Geometry: see drawing. Coordinates: mm, zero at the bounding-box minimum. A direction names the side the tool comes from. Give positions to 0.01 mm unless a question says otherwise; leave off trailing zeros. Loops run counter-clockwise (first coordinate to the right, second up) from the corner with the lowest first, then second, coordinate; pieces in that order, holes last. Notation, with made-up numbers: (-13, 81.25) -> (32, 81.25) arc R24 cw to (32, 99.25) -> close; hole circle Ø11 at (3.5, 56). An arc over 180 degrees is marked (long way). Return JSON: item names as keys, results as strings. Group by question number.
(1) Draft query along Y for the marked faces 3, 4, 5 and 6. Return one class per face: released by +Y, released by -Y, zero draft, split by the parting line, or undercut.
(2) Ray query, line 1 (Z direction, x = 25, y = 0.6); line 2 (X direction, y = 6, z = 10). Return the intervals inside material, ascending. Write a range as from..to.
(3) Pin query (flat end, axial travel): pin 1 (8 mm diameter, centred on y = 14.5, z = 18, fed in from +X); pin 2 (5.5 mm diameter, centred on x = 25, z = 21.25, fed in from -Y); pin 3 (12 mm diameter, centred on x = 4.5, y = 26, fed in from -Z); pin 4 (4.5 mm diameter, centred on x = 11, z = 21.25, fed in from +Y). Return the tip coordinate at first contact, or that it passes through.
(4) Cut plane B-B on x = 25. Return loops of the section in (y, z), then the cut area to 3 significant figures.
(5) Cut plane D-D on y = 17. Return loops of the section in (x, z), then the cut area to 3 significant figures.
(6) Cut plane A-A on z = 13.25. Return loops of the section in (x, y).
(7) Access query for the marked faces 1 and 2. Directions: +Z, -Z, +X, -X, +Y, -Y. A direction counts if a zero-diameter tool reaches every point of the face in a straight line with its end or side. Return the directions, or none.
(8) Cut plane C-C on x = 18. Return loops of the section in (y, z), then the cut area to 3 significant figures.
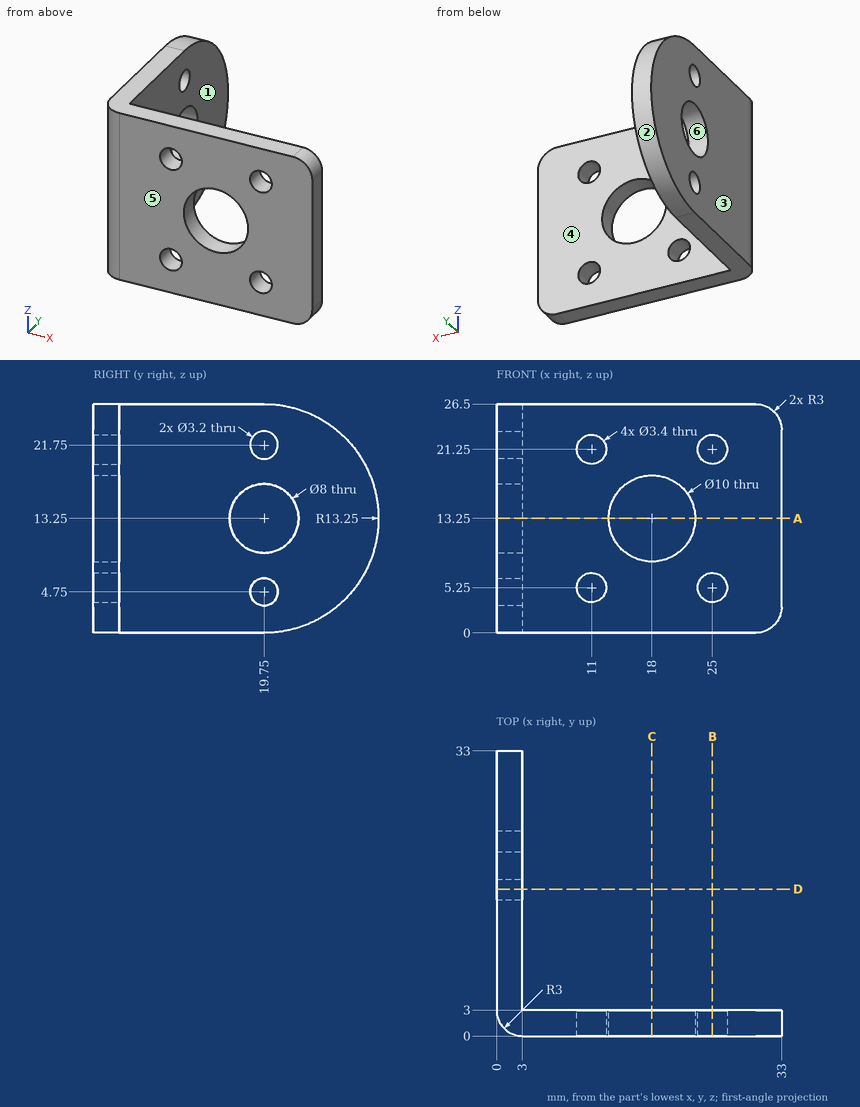
Answers:
{
 "1": {"face 3": "zero draft", "face 4": "released by +Y", "face 5": "released by -Y", "face 6": "undercut"},
 "2": {"line 1": "0..3.55, 6.95..19.55, 22.95..26.5", "line 2": "0..3"},
 "3": {"pin 1": "x = 3", "pin 2": "y = 0", "pin 3": "z = 0.01", "pin 4": "y = 3"},
 "4": {"outline": "(0, 0) -> (3, 0) -> (3, 3.55) -> (0, 3.55) -> close; (0, 6.95) -> (3, 6.95) -> (3, 19.55) -> (0, 19.55) -> close; (0, 22.95) -> (3, 22.95) -> (3, 26.5) -> (0, 26.5) -> close", "area": "59.1 mm²"},
 "5": {"outline": "(0, 0) -> (3, 0) -> (3, 10.35) -> (0, 10.35) -> close; (0, 16.15) -> (3, 16.15) -> (3, 26.5) -> (0, 26.5) -> close", "area": "62.1 mm²"},
 "6": {"outline": "(0, 3) arc R3 ccw to (3, 0) -> (13, 0) -> (13, 3) -> (3, 3) -> (3, 15.75) -> (0, 15.75) -> close; (0, 23.75) -> (3, 23.75) -> (3, 33) -> (0, 33) -> close; (23, 0) -> (33, 0) -> (33, 3) -> (23, 3) -> close"},
 "7": {"face 1": "+Z, -Z, +X, +Y", "face 2": "+X, -X, +Y"},
 "8": {"outline": "(0, 0) -> (3, 0) -> (3, 8.25) -> (0, 8.25) -> close; (0, 18.25) -> (3, 18.25) -> (3, 26.5) -> (0, 26.5) -> close", "area": "49.5 mm²"}
}
